The listing builds one solid part. Answer for the finished solid, in the listing's coordinates (mm). Face numbers are marked on the shaded views. A direction names the side the tool comes from. Round coordinates to 2 decimals unless told otherwise and drop trailing zeros. Order: outer loops, then holes, each group sorted by start corner. A loop starts at its lowest first (then second) coordinate and runs counter-clockwise, first axis right, second up. Notation, with made-up numbers: (-30, -10) - (0, -10) arc R23 ccw to (0, 13) - close; hole circle Ø3 at (76, 87.5). An arc over 180 degrees is marked (long way). Write item = value, one per line.
from build123d import *

# Parameters (mm, degrees)
EXTRUDE_1_DEPTH = 250
SKETCH_2_W      = 62
SKETCH_2_H      = 120
EXTRUDE_2_DEPTH = 60


with BuildPart() as part:
    # 草图1 → 凸台-拉伸1 (new body)
    with BuildSketch(Plane.XY):
        Polygon((-160, -160), (160, -160), (160, -42.368693821), (224.572052692, -42.368693821), (224.572052692, 160), (-160, 160), align=None)
        with BuildLine():
            Line((-140, 140), (140, 140))
            Line((140, 140), (140, 100))
            Line((140, 100), (202, 100))
            Line((202, 100), (202, -20))
            Line((202, -20), (140, -20))
            Line((140, -20), (140, -140))
            Line((140, -140), (-45, -140))
            ThreePointArc((-45, -140), (-72.824855787, -72.824855787), (-140, -45))
            Line((-140, -45), (-140, 140))
        make_face(mode=Mode.SUBTRACT)
    extrude(amount=EXTRUDE_1_DEPTH)

    # 草图2 → 凸台-拉伸2 (add)
    with BuildSketch(Plane(origin=(0, 0, 0), x_dir=(-1, 0, 0), z_dir=(0, 0, -1))):
        with Locations((-171, 40)):
            Rectangle(SKETCH_2_W, SKETCH_2_H)
    extrude(amount=-EXTRUDE_2_DEPTH)


solid = part.part
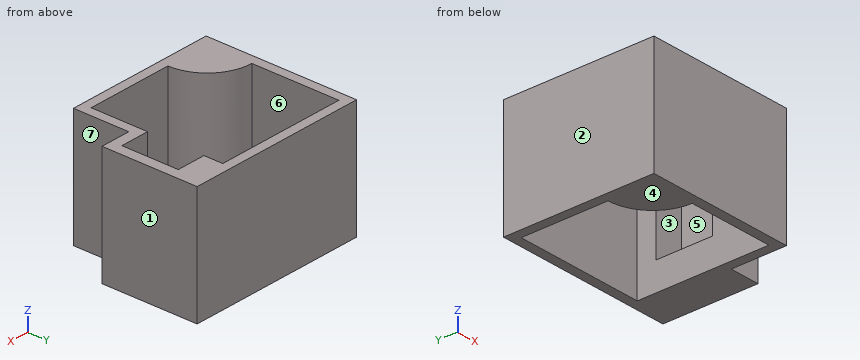
Q1. Section A-A on y = 43.5 is taken. Determine the outline of the cut face in (x, z), then the cut area to 3 significant figures.
Model answer:
outline = (-160, 0) - (-140, 0) - (-140, 250) - (-160, 250) - close; (140, 0) - (224.57, 0) - (224.57, 250) - (202, 250) - (202, 60) - (140, 60) - close
area = 14,400 mm^2
Q2. Flat-ended cylindrical pins translate along their axes: P1, Ø18.5, axis at x = 163.5, y = 69.5, coming from the +Z side; P2, Ø18.5, axis at x = 172, z = 151.5, coming from the -Y side. Find the tip coordinate at first contact, or state that the pin passes through.
Model answer:
P1 = 60
P2 = -42.37
Q3. For the marked faces 4, 5, 6 and 7, determine the directions among +Z, -Z, +X, -X, +Y, -Y from which every point of the face is accessible in a straight line to the end or side of a thin tool.
Model answer:
face_4 = -Z, +X, -X, +Y, -Y
face_5 = +Z
face_6 = +Z, -Z
face_7 = +Z, -Z, +X, -Y
Q4. Determine the mould class of the marked faces 1, 2 and 3 for opening direction X: released by +X, released by -X, zero draft, split by the parting line, or undercut.
Model answer:
face_1 = released by +X
face_2 = released by -X
face_3 = undercut
Q5. Section C-C on z = 227 is taken. Determine the outline of the cut face in (x, y), then the cut area to 3 significant figures.
Model answer:
outline = (-160, -160) - (160, -160) - (160, -42.37) - (224.57, -42.37) - (224.57, 160) - (-160, 160) - close; hole (-140, -45) arc R95 cw to (-45, -140) - (140, -140) - (140, -20) - (202, -20) - (202, 100) - (140, 100) - (140, 140) - (-140, 140) - close
area = 36,700 mm^2
Q6. Section B-B on x = 77.5 is taken. Determine the outline of the cut face in (y, z), then the cut area to 3 significant figures.
Model answer:
outline = (-160, 0) - (-140, 0) - (-140, 250) - (-160, 250) - close; (140, 0) - (160, 0) - (160, 250) - (140, 250) - close
area = 10,000 mm^2
Q7. Section D-D on x = 177 is taken. Determine the outline of the cut face in (y, z).
Model answer:
outline = (-42.37, 0) - (160, 0) - (160, 250) - (100, 250) - (100, 60) - (-20, 60) - (-20, 250) - (-42.37, 250) - close
Q8. Find the intervals of material crossed by line 1 (Y direction, x = 162, z = 100.5); line 2 (Y direction, x = -26.5, z = 145); line 3 (X direction, y = 95, z = 236), in increasing order. Write a range as from..to.
Model answer:
line_1 = -42.37..-20, 100..160
line_2 = -160..-140, 140..160
line_3 = -160..-140, 202..224.57
